Read the model definition and answer for the solid it produces. Units are mm, in the model's axes. A direction names the side the tool comes from. Coordinates: 2 decimals unless noted, no trailing zeros. Loops run counter-clockwise (first coordinate to the right, second up) from the corner with the lowest first, then second, coordinate; pieces in that order, holes last. Notation, with made-up numbers: (45, -21) -> (62, -21) arc R26 ccw to (62, 14) -> close; hole circle Ø7 at (-12, 20.25). An arc over 180 degrees is marked (long way). One line per question, with ' | ' between items. Start each with the question number.
Autodesk Inventor part; units mm, degrees
ref_plane "YZ Plane" through (0, 0, 0) normal (1, 0, 0) x (0, 1, 0)
ref_plane "XZ Plane" through (0, 0, 0) normal (0, 1, 0) x (-1, 0, 0)
ref_plane "XY Plane" through (0, 0, 0) normal (0, 0, 1) x (1, 0, 0)
sketch "Sketch1" plane through (0, 0, 0) normal (0, 1, 0) x (-1, 0, 0)
  line L0 (-17.05, 0) -> (-17.05, 8.4971)
  line L1 (-17.05, 0) -> (-17.05, -8.4971)
  line L2 (17.05, 0) -> (17.05, 8.4971)
  line L3 (17.05, 0) -> (17.05, -8.4971)
  arc A0 (-17.05, -8.4971) -> (17.05, -8.4971) centre (0, 0) ccw
  arc A1 (17.05, 8.4971) -> (-17.05, 8.4971) centre (0, 0) ccw
extrude "Extrusion1" add sketch "Sketch1" along normal blind 3.175
sketch "Sketch4" plane through (0, 0, 0) normal (0, -1, 0) x (-1, 0, 0)
  line L0 (-13.4937, -0.7938) -> (13.4938, -0.7938)
  line L1 (13.4938, -0.7938) -> (13.4938, 0.7938)
  line L2 (13.4938, 0.7938) -> (-13.4938, 0.7937)
  line L3 (-13.4938, 0.7937) -> (-13.4937, -0.7938)
  circle A0 centre (0, 0) radius 19.05
  dimension "d16" = 26.9875
  dimension "d17" = 1.5875
  dimension "d18" = 18.2563
  dimension "d19" = 5.5563
extrude "Extrusion3" add sketch "Sketch4" along normal blind 12.7 contours L3 L2 L1 L0
sketch "Sketch5" plane through (0, 0, 0) normal (0, -1, 0) x (-1, 0, 0)
  line L0 (13.4937, 0.7938) -> (-13.4938, 0.7937)
  line L1 (-0.7938, 0.7937) -> (0.6758, 0.7937)
  line L2 (0.6758, 0.7937) -> (0.6758, 13.4938)
  line L3 (0.6758, 13.4938) -> (-0.7938, 13.4938)
  line L4 (-0.7938, 13.4938) -> (-0.7938, 0.7937)
  line L5 (-13.4938, 0.7937) -> (-13.4937, -0.7938)
  point P0 (0, 0)
  dimension "d22" = 12.7
  dimension "d23" = 12.7
extrude "Extrusion4" add sketch "Sketch5" along normal blind 12.7
sketch "Sketch7" plane through (0, 0, 0) normal (0, -1, 0) x (-1, 0, 0)
  line L0 (-13.4937, -0.7938) -> (13.4937, -0.7938)
  line L1 (-0.7938, -0.7938) -> (0.7937, -0.7938)
  line L2 (0.7937, -0.7938) -> (0.7937, -13.4938)
  line L3 (0.7937, -13.4938) -> (-0.7938, -13.4938)
  line L4 (-0.7938, -13.4938) -> (-0.7938, -0.7938)
  line L5 (13.4937, -0.7938) -> (13.4937, 0.7938)
  point P0 (0, 0)
  dimension "d28" = 12.7
  dimension "d29" = 1.5875
  dimension "d30" = 12.7
extrude "Extrusion5" add sketch "Sketch7" along normal blind 12.7
properties part number "Syringe cap_Flat_Sides"
(1) Section D-D on y = 1.25 is taken. Write down the section's boundary in (x, z).
(2) Section C-C on x = 0 is taken. Write down the section's boundary in (y, z) (3 decimals).
(3) Each of these flat-tipped pins is pushed along its axis until it touches: pin 1 Ø4 at (x, y) = (-8.5, -7.5) entering from +Z; pin 2 Ø0.7 at (x, y) = (0.5, -6) entering from -Z; pin 3 Ø1.5 at (y, z) = (-8.5, 12) entering from +X. Where does it stop, or does it pass through?
(4) Section A-A on y = -11.5 is taken. Write down the section's boundary in (x, z), plus the area to 3 significant figures.
(5) Find the intervals of material crossed by probe 1 along Z at (x, y) = (8, -2.75); probe 2 along Y at (x, z) = (4, -4) (3 decimals), in increasing order. Write a range as from..to.
(6) Section B-B on z = -7 is taken. Write down the section's boundary in (x, y) (3 decimals).
(7) A tool of negligible diameter and unlimited length cuts with its end or side. For faces 1 (the flat face through (7, -6, 0.794)), 2 (the flat face through (0.794, -6, -7)), 3 (the flat face through (0, -6, 13.494)), from which of +Z, -Z, +X, -X, +Y, -Y can it reach the whole face along a straight path? Write none if from no direction.
Working result:
1) outline: (-17.05, -8.5) arc R19.05 ccw to (17.05, -8.5) -> (17.05, 8.5) arc R19.05 ccw to (-17.05, 8.5) -> close
2) outline: (-12.7, -13.494) -> (0, -13.494) -> (0, -19.05) -> (3.175, -19.05) -> (3.175, 19.05) -> (0, 19.05) -> (0, 13.494) -> (-12.7, 13.494) -> close
3) pin 1: stops at z = 0.79 | pin 2: stops at z = -13.49 | pin 3: stops at x = 0.79
4) outline: (-13.49, -0.79) -> (-0.68, -0.79) -> (-0.68, -13.49) -> (0.79, -13.49) -> (0.79, -0.79) -> (13.49, -0.79) -> (13.49, 0.79) -> (0.79, 0.79) -> (0.79, 13.49) -> (-0.79, 13.49) -> (-0.79, 0.79) -> (-13.49, 0.79) -> close | area: 81.7 mm2
5) probe 1: z = -0.79..0.79 | probe 2: y = 0..3.175
6) outline: (-17.05, 0) -> (-0.676, 0) -> (-0.676, -12.7) -> (0.794, -12.7) -> (0.794, 0) -> (17.05, 0) -> (17.05, 3.175) -> (-17.05, 3.175) -> close
7) face 1: +Z, +X, -Y | face 2: -Z, +X, -Y | face 3: +Z, +X, -X, -Y
